Here's how the part is built. I have some questions about the finished solid (model axes, mm). Face numbers are marked on the shaded views. A direction names the side the tool comes from. Round coordinates to 2 decimals unless told otherwise and drop trailing zeros. Loops run counter-clockwise (first coordinate to the right, second up) from the corner with the lowest first, then second, coordinate; pieces in that order, holes last. Notation, with made-up numbers: (58.5, -24) - (73.5, -24) arc R8 ccw to (73.5, -15) - close; hole circle Ø6 at (70.25, 35.25). An arc over 180 degrees is marked (long way). Return JSON: item names as keys, results as strings. Group by question number.
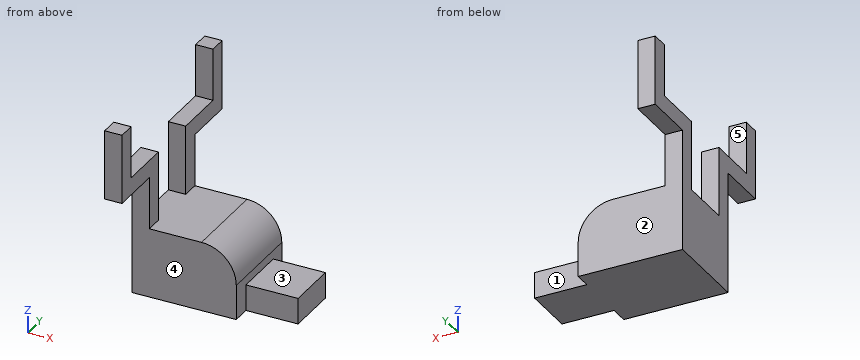
```python
from build123d import *

# Parameters (mm, degrees)
F0_W      = 30
F0_H      = 25
F1_DEPTH  = 20
F2_W      = 15
F2_H      = 7.5
F3_DEPTH  = 15
F4_W      = 5
F4_H      = 5
F5_DEPTH  = 20
F6_W      = 5
F6_H      = 5
F7_DEPTH  = 15
F8_W      = 5
F8_H      = 5
F9_DEPTH  = 15
F10_W     = 5
F10_H     = 5
F11_W     = 5
F11_H     = 5
F12_DEPTH = 15
F13_R     = 10


with BuildPart() as f1:
    # F0 (on Top) → F1 (new body)
    with BuildSketch(Plane.XY):
        with Locations((-42.374329, -29.235112)):
            Rectangle(F0_W, F0_H)
    extrude(amount=F1_DEPTH)

    # F2 (on face) → F3 (join)
    with BuildSketch(Plane.YZ.offset(-27.374329)):
        with Locations((-28.950002, 3.75)):
            Rectangle(F2_W, F2_H)
    extrude(amount=F3_DEPTH)

    # F4 (on face) → F5 (join)
    with BuildSketch(Plane.XY.offset(20)):
        with Locations((-54.874329, -19.235112)):
            Rectangle(F4_W, F4_H)
        with Locations((-54.874329, -39.235112)):
            Rectangle(F4_W, F4_H)
    extrude(amount=F5_DEPTH)

    # F6 (on face) → F7 (join)
    with BuildSketch(Plane(origin=(0, -16.735112, 0), x_dir=(-1, 0, 0), z_dir=(0, 1, 0))):
        with Locations((54.874329, 37.5)):
            Rectangle(F6_W, F6_H)
    extrude(amount=F7_DEPTH)

    # F8 (on face) → F9 (join)
    with BuildSketch(Plane.XZ.offset(41.735112)):
        with Locations((-54.874329, 37.5)):
            Rectangle(F8_W, F8_H)
    extrude(amount=F9_DEPTH)

    # F10 (on face) + F11 (on face) → F12 (join)
    with BuildSketch(Plane.XY.offset(40)):
        with Locations((-54.874329, -4.235112)):
            Rectangle(F10_W, F10_H)
    with BuildSketch(Plane.XY.offset(40)):
        with Locations((-54.874329, -54.235112)):
            Rectangle(F11_W, F11_H)
    extrude(amount=F12_DEPTH)

    # F13
    f13_edges = [f1.edges().sort_by_distance(p)[0] for p in [
        (-27.374329, -29.235112, 20),
    ]]
    fillet(f13_edges, radius=F13_R)


solid = f1.part
```
Q1. Imagine slicing it at A-A, the plane z = 32.5. List the corners of the cut face in (x, y) for me.
Q2. For the marked faces 1, 2, 3, 4 and 5, which set-ups out of +Z, -Z, +X, -X, +Y, -Y let a thin tool reach every point of the face, with its end or its side?
Q3. Imagine slicing it at B-B, the plane y = -41. List the corners of the cut face in (x, z) for me, and give its area (3 significant figures).
Q4. Imagine slicing it at C-C, the plane z = 5.5. List the corners of the cut face in (x, y) for me.
Q5. Please list where these lines run through material, in increasing order: line 1 (Y direction, x = -53.5, z = 3); line 2 (Z direction, x = -44, y = -40); line 3 (X direction, y = -41, z = 32).
Q6. Imagine slicing it at D-D, the plane x = -43. List the corners of the cut face in (y, z) for me.
Q7. Will these pins go through, and if not, where does the flat tip stop? pin 1 Ø1.5 at (x, z) = (-30, 5.5) entering from -Y; pin 2 Ø12 at (x, y) = (-16.5, -25.5) entering from +Z; pin 3 Ø2.5 at (x, y) = (-53.5, -43) entering from +Z.
Output values:
{
 "1": {"outline": "(-57.37, -41.74) - (-52.37, -41.74) - (-52.37, -36.74) - (-57.37, -36.74) - close; (-57.37, -21.74) - (-52.37, -21.74) - (-52.37, -16.74) - (-57.37, -16.74) - close"},
 "2": {"face 1": "+Z, -Z, +X, +Y", "face 2": "-Z, +X, -X, +Y", "face 3": "+Z, +X, +Y, -Y", "face 4": "-Z, +X, -X, -Y", "face 5": "+Z, +X, -X"},
 "3": {"outline": "(-57.37, 0) - (-27.37, 0) - (-27.37, 10) arc R10 ccw to (-37.37, 20) - (-52.37, 20) - (-52.37, 40) - (-57.37, 40) - close", "area": "679 mm^2"},
 "4": {"outline": "(-57.37, -41.74) - (-27.37, -41.74) - (-27.37, -36.45) - (-12.37, -36.45) - (-12.37, -21.45) - (-27.37, -21.45) - (-27.37, -16.74) - (-57.37, -16.74) - close"},
 "5": {"line 1": "y = -41.74 to -16.74", "line 2": "z = 0 to 20", "line 3": "x = -57.37 to -52.37"},
 "6": {"outline": "(-41.74, 0) - (-16.74, 0) - (-16.74, 20) - (-41.74, 20) - close"},
 "7": {"pin 1": "stops at y = -41.74", "pin 2": "stops at z = 7.5", "pin 3": "stops at z = 40"}
}
